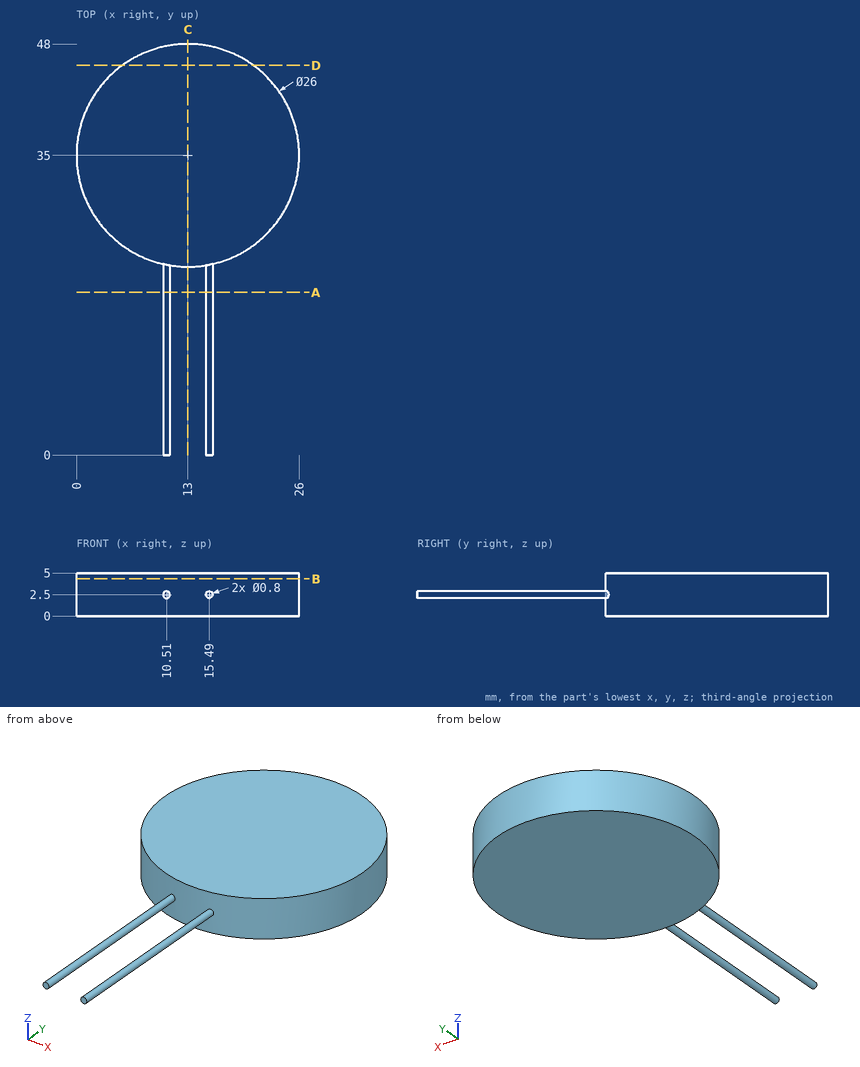
Study the drawing (mm; zero at the part's minimum x, y, z) and answer. Give positions to 0.01 mm unless a question says otherwise; leave off trailing zeros. Order: outer loops, then holes, each group sorted by start corner. A loop starts at its lowest first (then second) coordinate and runs counter-clockwise, first axis right, second up. Notation, with made-up numbers: (-26.75, -35) - (-19.75, -35) arc R15 cw to (-19.75, -21) - close; hole circle Ø6 at (-40, 23.25). An arc over 180 degrees is marked (long way). Answer in a Markdown table with one row per item. Add a question column.
Q1. The part is cut by section C-C (x = 13). Determine the outline of the cut face in (y, z), then the cut area to 3 significant figures.
Q2. Given P1, Ø3, axis at x = 9, z = 1, coming from the +Y side; P2, Ø3, axis at x = 3, y = 25.5, coming from the +Z side; P3, Ø3, axis at x = 19, z = 3.5, coming from the -Y side; P4, Ø1, axis at x = 7.5, z = 4.5, coming from the +Y side, each flat-ended and moving along its own axis, determine where each tip first touches the part or whether it passes through.
Q3. The part is cut by section D-D (y = 45.5). Determine the outline of the cut face in (x, z) (1 decimal).
Q4. The part is cut by section A-A (y = 19). Determine the outline of the cut face in (x, z).
Q5. The part is cut by section B-B (z = 4.35). Determine the outline of the cut face in (x, y).
Q6. Find the intervals of material crossed by line 1 along X through (y, z) = (3.5, 2.3) (1 decimal); line 2 along X through (y, z) = (44, 3.9); line 3 along Y through (x, z) = (5.75, 0.7), in increasing order. Write a range as [from, to].
Determined:
| question | item | result |
|---|---|---|
| 1 | outline | (22, 0) - (48, 0) - (48, 5) - (22, 5) - close |
| 1 | area | 130 mm² |
| 2 | P1 | stops at y = 47.76 |
| 2 | P2 | stops at z = 5 |
| 2 | P3 | stops at y = 22.8 |
| 2 | P4 | stops at y = 47 |
| 3 | outline | (5.3, 0) - (20.7, 0) - (20.7, 5) - (5.3, 5) - close |
| 4 | outline | circle Ø0.8 at (10.51, 2.5); circle Ø0.8 at (15.49, 2.5) |
| 5 | outline | circle Ø26 at (13, 35) |
| 6 | line 1 | x = [10.2, 10.9], [15.1, 15.8] |
| 6 | line 2 | x = [3.62, 22.38] |
| 6 | line 3 | y = [24.21, 45.79] |
